Autodesk Fusion 360 part; units mm, degrees
sketch "Sketch1" plane through (0, 0, 0) normal (0, 1, 0) x (1, 0, 0)
  line L0 (0, 0) -> (-37.75, 0)
  line L1 (-37.75, 0) -> (-40.6618, -8)
  line L2 (-40.6618, -8) -> (-39.0618, -8)
  line L3 (-39.0618, -8) -> (-36.95, -3.5)
  line L4 (-36.95, -3.5) -> (-37.75, -3.5)
  line L5 (-37.75, -3.5) -> (-37.75, -1.6)
  line L6 (-37.75, -1.6) -> (0, -1.6)
  line L7 (0, -1.6) -> (0, 0)
  line L8 (0, -1.6) -> (0, -8)
  line L9 (-39.0239, -3.5) -> (-39.0239, 0)
  line L10 (-39.0239, 0) -> (-37.75, 0)
  dimension "d1" = 75.5
  dimension "d2" = 1.6
  dimension "d3" = 0.8
  dimension "d4" = 1.9
  dimension "d5" = 8
  dimension "d6" = 1.6
  dimension "d7" = 110
  dimension "d9" = 75.5
revolve "Revolve1" add sketch "Sketch1" angle 360 about axis through (0, 0, 1.6) along (0, 0, 1)
chamfer "Chamfer1" distance 0.2 angle 45 1 edges at (-35.1954, 13.651, 1.6)
chamfer "Chamfer2" distance 0.7 distance2 0.4 1 edges at (-35.1954, 13.651, 3.5) measured on face at (11.897, 35.4466, 3.5)
chamfer "Chamfer3" distance 0.4 distance2 0.4 2 edges at (-36.4183, 14.1253, 8) (-37.9101, 14.7039, 8) measured on face at (-39.8316, 3.9607, 8) measured on face at (-39.9165, 3.9942, 6.5)
chamfer "Chamfer4" distance 0.4 distance2 0.4 1 edges at (-36.383, 14.1116, 0) measured on face at (0.5395, 14.867, 0)
equation "d1 = Linear Dimension-2"
equation "d2 = Linear Dimension-3"
equation "d3 = Linear Dimension-4"
equation "d4 = Linear Dimension-5"
equation "d5 = height"
equation "d6 = Linear Dimension-7"
equation "d9 = Linear Dimension-9"
equation "height = 8 mm"
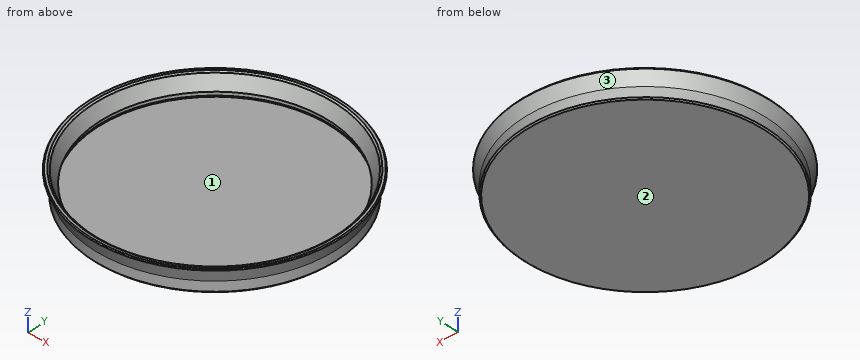
Source: CAD feature listing. Evaluate the final solid. Frame: model axes, mm. Face numbers are marked on the shaded views. Give positions to 0.01 mm unless a question says otherwise; leave off trailing zeros. Loops run counter-clockwise (first coordinate to the right, second up) from the corner with the lowest first, then second, coordinate; pieces in that order, holes last. Notation, with made-up numbers: (65.5, 66.5) - (101.5, 66.5) arc R20 ccw to (101.5, 76.5) - close; hole circle Ø3 at (-39, -28.75). An arc over 180 degrees is marked (long way). Use CSV: the item, a comma, the result in double quotes.
1) Pin query (flat end, axial travel): P1, Ø12, axis at x = -24.5, y = -28, coming from the -Z side; P2, Ø1.5, axis at x = -7, z = 5, coming from the +Y side; P3, Ø1.5, axis at y = -18.5, z = 6.5, coming from the +X side; P4, Ø1, axis at x = -30, z = 3, coming from the +Y side. Return the tip coordinate at first contact, or that it passes through.
Worked out:
P1,"stops at z = 0"
P2,"stops at y = 39.25"
P3,"stops at x = 36.08"
P4,"stops at y = 25.55"
2) Line query: line 1 (X direction, y = 0, z = 2.6); line 2 (Z direction, x = -22, y = -25). Output: solid intervals per line, ascending.
Worked out:
line 1,"x = -39.02 to -37.75, 37.75 to 39.02"
line 2,"z = 0 to 1.6"
3) Cut plane A-A (y = 0). Output: boundary loops of the cut face in (x, z) (3 decimals), and give its area (3 significant figures).
Worked out:
outline,"(-40.525, 7.624) - (-39.024, 3.5) - (-39.024, 0.4) - (-38.624, 0) - (38.624, 0) - (39.024, 0.4) - (39.024, 3.5) - (40.525, 7.624) - (40.262, 8) - (39.462, 8) - (38.892, 7.638) - (36.95, 3.5) - (37.05, 3.5) - (37.75, 3.1) - (37.75, 1.8) - (37.55, 1.6) - (-37.55, 1.6) - (-37.75, 1.8) - (-37.75, 3.1) - (-37.05, 3.5) - (-36.95, 3.5) - (-38.892, 7.638) - (-39.462, 8) - (-40.262, 8) - close"
area,"146 mm^2"
4) Cut plane C-C (z = 5.5). Output: boundary loops of the cut face in (x, y), and give its area (3 significant figures).
Worked out:
outline,"circle Ø79.5 at (0, 0); hole circle Ø75.78 at (0, 0)"
area,"454 mm^2"
5) Mould query, pull axis Y, two halves, no side actions, for the marked faces 1, 2 and 3. Classes: +Y half, -Y half, draft (parallel to the pull), parting line (faces both ways), or undercut.
Worked out:
face 1,"undercut"
face 2,"draft"
face 3,"parting line"
